Here's how the part is built. I have some questions about the finished solid (model axes, mm). A direction names the side the tool comes from. Round coordinates to 2 decimals unless told otherwise and drop trailing zeros. Answer as CSV lines item,"result".
Autodesk Inventor part; units mm, degrees
ref_plane "YZ Plane" through (0, 0, 0) normal (1, 0, 0) x (0, 1, 0)
ref_plane "XZ Plane" through (0, 0, 0) normal (0, 1, 0) x (-1, 0, 0)
ref_plane "XY Plane" through (0, 0, 0) normal (0, 0, 1) x (1, 0, 0)
sketch "Sketch1" plane through (0, 0, 0) normal (0, 0, 1) x (1, 0, 0)
  line L0 (111.25, 0) -> (-111.25, 0) construction
  line L1 (111.25, 33.4225) -> (-111.25, 33.4225) construction
  line L2 (-111.25, -33.4225) -> (111.25, -33.4225) construction
  arc A0 (111.25, -33.4225) -> (111.25, 33.4225) centre (111.25, 0) ccw construction
  arc A1 (-111.25, 33.4225) -> (-111.25, -33.4225) centre (-111.25, 0) ccw construction
  line L3 (-111.25, 35.7085) -> (111.25, 35.7085)
  arc A2 (111.25, -35.7085) -> (111.25, 35.7085) centre (111.25, 0) ccw
  line L4 (111.25, -35.7085) -> (-111.25, -35.7085)
  arc A3 (-111.25, 35.7085) -> (-111.25, -35.7085) centre (-111.25, 0) ccw
  line L5 (-111.25, 31.835) -> (111.25, 31.835)
  arc A4 (111.25, -31.835) -> (111.25, 31.835) centre (111.25, 0) ccw
  line L6 (111.25, -31.835) -> (-111.25, -31.835)
  arc A5 (-111.25, 31.835) -> (-111.25, -31.835) centre (-111.25, 0) ccw
  point P0 (0, 0)
  dimension "d0" = 66.8451
  dimension "d1" = 105
  dimension "d2" = 222.5
  dimension "d3" = 2.286
  dimension "d4" = 1.5875
extrude "Extrusion1" add sketch "Sketch1" along normal mid plane 15
fillet "Fillet1" radius 0.254 8 edges at (0, 35.7085, 7.5) (-146.9585, 0, 7.5) (0, -35.7085, 7.5) (146.9585, 0, 7.5) (146.9585, 0, -7.5) (0, -35.7085, -7.5) (-146.9585, 0, -7.5) (0, 35.7085, -7.5)
properties part number "Configurable Kitbot Drive Belt" material "Rubber"
Item 1: If we mould it in two halves opening along Y, with no side actions, what happens to faces 1 (the cylindrical face through (-143.077, -0.7, -0.105)), 2 (the cylindrical face through (146.95, 0.79, -0.1)), 3 (the flat face through (2, -31.835, 0)), 4 (the flat face through (-1, -34, -7.5))? For each: pulls with the +Y half, pulls with the -Y half, needs draft (parallel to the pull), parting line crosses it, or undercut.
Results found:
face 1,"undercut"
face 2,"parting line crosses it"
face 3,"undercut"
face 4,"needs draft"
Item 2: I need wall thicknesses on L1, parallel to Y at x = -57, z = 6.75 (1 decimal); L2, parallel to Y at x = -130, z = 3; L3, parallel to X at y = -10, z = -5.25. Which ranges of each line are inside material? Lowest first, please.
Results found:
L1,"y = -35.7 to -31.8, 31.8 to 35.7"
L2,"y = -30.39 to -25.73, 25.73 to 30.39"
L3,"x = -145.53 to -141.47, 141.47 to 145.53"
Item 3: Will these pins go through, and if not, where does the flat tip stop? pin 1 (1 mm diameter, centred on y = 26.5, z = -0.5, fed in from +X); pin 2 (2 mm diameter, centred on y = 1.5, z = 3, fed in from -X) (3 decimals).
Results found:
pin 1,"stops at x = 135.73"
pin 2,"stops at x = -146.955"
Item 4: For faces 5 (the flat face through (2, -35.708, 0)), 6 (the flat face through (-2, 31.835, 0)), which set-ups out of +Z, -Z, +X, -X, +Y, -Y let a thin tool reach every point of the face, with its end or its side?
Results found:
face 5,"+Z, -Z, +X, -X, -Y"
face 6,"+Z, -Z"
